The listing builds one solid part. Answer for the finished solid, in the listing's coordinates (mm). A direction names the side the tool comes from. Round coordinates to 2 decimals unless told otherwise and drop trailing zeros. Order: outer loops, then holes, each group sorted by start corner. A loop starts at its lowest first (then second) coordinate and runs counter-clockwise, first axis right, second up. Notation, with made-up numbers: (82, 63.25) - (108, 63.25) arc R30 cw to (108, 87.25) - close; hole circle Ø9 at (-21, -19). An arc over 180 degrees is marked (long way). Use CSV: the item, a comma, the result in double quotes. Start each with the question number.
Item 1: Find section B-B, the plane z = -1. Give the vertices of the cut face in (x, y), plus the area to 3 significant figures.
Item 2: Flat-ended cylindrical pins translate along their axes: P1, Ø4, axis at x = -7.5, z = -3, coming from the +Y side; P2, Ø3.5, axis at y = 0.5, z = -7.5, coming from the -X side; P3, Ø4, axis at x = -7.5, z = -2, coming from the -Y side. Find the tip coordinate at first contact, or state that the pin passes through.
Item 3: Find section A-A, the plane z = -5.75. Give the vertices of the cut face in (x, y).
Item 4: For faces 1 (the flat face through (3.2, -5.66, -6.7)), 2 (the flat face through (-6.5, 0, -7)), 3 (the cylindrical face through (-1.73, 7.81, -3.25)), determine the directions among +Z, -Z, +X, -X, +Y, -Y from which every point of the face is accessible in a straight line to the end or side of a thin tool.
Item 5: Straight lines are drawn through the part: line 1 along Z through (x, y) = (7.5, -2); line 2 along X through (y, z) = (-0.5, -5.25); line 3 along Y through (x, z) = (3.25, -6.25). For each, find the intervals that lie inside material, in ascending order. Write a range as [from, to].
Item 6: Determine the mould class of faces 4 (the flat face through (0, 5, 0)), 5 (the conical face through (-1.8, 8, -2.9)), 6 (the cylindrical face through (-0.867, -3.905, -4.93)) for opening direction X: +X half, -X half, draft (parallel to the pull), parting line (faces both ways), or undercut.
```python
from build123d import *

# Parameters (mm, degrees)
BASE_EXTRUSION_DEPTH    = 10
ESQUISSE3_R             = 4
ENL_V_MAT_EXTRU_1_DEPTH = 15.091959883


with BuildPart() as part:
    # Esquisse1 → Base-Extrusion (new body)
    with BuildSketch(Plane.XY):
        Polygon((6.5, -3.75277675), (6.5, 3.75277675), (0, 7.505553499), (-6.5, 3.75277675), (-6.5, -3.75277675), (0, -7.505553499), align=None)
    extrude(amount=-BASE_EXTRUSION_DEPTH)

    # Esquisse2 → Enl_vement de mati_re-R_volution1 (revolve, cut)
    with BuildSketch(Plane(origin=(0, 0, 0), x_dir=(1, 0, 0), z_dir=(0, 1, 0)), mode=Mode.PRIVATE) as enl_vement_de_mati_re_r_volution1_sk:
        Polygon((-6.5, 10), (-23.820508076, 10), (-23.820508076, 0), align=None)
    revolve(enl_vement_de_mati_re_r_volution1_sk.sketch.rotate(Axis((0, 0, -10), (0, 0, 1)), 180), axis=Axis((0, 0, -10), (0, 0, 1)), mode=Mode.SUBTRACT)

    # Esquisse3 → Enl_v. mat.-Extru.1 (cut, through all)
    with BuildSketch(Plane.XY):
        Circle(ESQUISSE3_R)
    extrude(amount=-ENL_V_MAT_EXTRU_1_DEPTH, mode=Mode.SUBTRACT)

    # Esquisse4 → Boss.-R_vol.1 (revolve)
    with BuildSketch(Plane(origin=(0, 0, 0), x_dir=(1, 0, 0), z_dir=(0, 1, 0)), mode=Mode.PRIVATE) as boss_r_vol_1_sk:
        Polygon((-6.5, 0), (-11, 0), (-11, 1.5), (-8, 3), (-8, 3.5), (-6.5, 3.5), align=None)
    revolve(boss_r_vol_1_sk.sketch.rotate(Axis((0, 0, 0), (0, 0, -1)), 180), axis=Axis((0, 0, 0), (0, 0, -1)))


solid = part.part
```
Worked out:
1,outline,"circle Ø22 at (0, 0); hole circle Ø8 at (0, 0)"
1,area,"330 mm²"
2,P1,"stops at y = 9.1"
2,P2,"stops at x = -6.5"
2,P3,"stops at y = -9.49"
3,outline,"(-6.5, -3.75) - (0, -7.51) - (6.5, -3.75) - (6.5, 3.75) - (0, 7.51) - (-6.5, 3.75) - close; hole circle Ø8 at (0, 0)"
4,face 1,"-Z, +X, -Y"
4,face 2,"-Z, -X, +Y, -Y"
4,face 3,"-Z"
5,line 1,"z = [-3.5, 0]"
5,line 2,"x = [-6.5, -3.97], [3.97, 6.5]"
5,line 3,"y = [-5.63, -2.33], [2.33, 5.63]"
6,face 4,"draft"
6,face 5,"parting line"
6,face 6,"undercut"
